The listing builds one solid part. Answer for the finished solid, in the listing's coordinates (mm). Round coordinates to 2 decimals unless told otherwise and drop trailing zeros. Order: outer loops, then holes, each group sorted by start corner. A loop starts at its lowest first (then second) coordinate and runs counter-clockwise, first axis right, second up. Notation, with made-up numbers: M 71.5,-27.75 L 80.5,-27.75 A12 ccw 80.5,-17.75 Z; hole C 21,1.5 d5. An arc over 180 degrees is marked long. Write item = value, one per line. Start each with the question number.
(1) For a pull along X with two mould halves and no side action, classify faces 1 (the face through (-1.72, 1.61, 7.76)), 2 (the face through (0, 2, -16.51)), 3 (the face through (-19.85, 1.565, -15.746)) as released by +X, released by -X, zero draft, split by the parting line, or undercut.
(2) A cutting plane is placed at A-A, the plane y = 1.8. Determine the outline of the cut face in (x, z).
(3) Straight lines are drawn through the part: probe 1 along Z at (x, y) = (0, 1.6); probe 2 along X at (y, z) = (0.7, 0); probe 3 along X at (y, z) = (1.1, -4). For each, find the intervals that lie inside material, in ascending order. Write a range as from..to.
(4) This flat-tipped pin is pushed along its axis until it touches: pin 1 (9.5 mm diameter, centred on x = 0, z = 0, fed in from -Y). Where does it stop, or does it pass through?
(5) A cutting plane is placed at B-B, the plane z = 0. Determine the outline of the cut face in (x, y) (3 decimals), and give its area (3 significant figures).
(6) A cutting plane is placed at C-C, the plane x = 0. Determine the outline of the cut face in (y, z) (3 decimals), and give its area (3 significant figures).
from build123d import *

# Parameters (mm, degrees)
BOSS_EXTRUDE1_DEPTH = 3.175
SKETCH2_R           = 7.9502
CUT_EXTRUDE1_DEPTH  = 4.175


with BuildPart() as part:
    # Sketch1 → Boss-Extrude1 (new body)
    with BuildSketch(Plane(origin=(0, 0, 0), x_dir=(1, 0, 0), z_dir=(0, 1, 0))):
        with BuildLine():
            Line((18.034, -16.51), (-18.034, -16.51))
            ThreePointArc((-18.034, -16.51), (-19.830051224, -15.766051224), (-20.574, -13.97))
            Line((-20.574, -13.97), (-20.574, 13.97))
            ThreePointArc((-20.574, 13.97), (-19.830051224, 15.766051224), (-18.034, 16.51))
            Line((-18.034, 16.51), (18.034, 16.51))
            ThreePointArc((18.034, 16.51), (19.830051224, 15.766051224), (20.574, 13.97))
            Line((20.574, 13.97), (20.574, -13.97))
            ThreePointArc((20.574, -13.97), (19.830051224, -15.766051224), (18.034, -16.51))
        make_face()
    extrude(amount=BOSS_EXTRUDE1_DEPTH)

    # Sketch2 → Cut-Extrude1 (cut, through all)
    with BuildSketch(Plane(origin=(0, 3.175, 0), x_dir=(1, 0, 0), z_dir=(0, 1, 0))):
        Circle(SKETCH2_R)
    extrude(amount=-CUT_EXTRUDE1_DEPTH, mode=Mode.SUBTRACT)


solid = part.part
Reported:
q1.face_1 = undercut
q1.face_2 = zero draft
q1.face_3 = released by -X
q2.outline = M -20.57,-13.97 A2.54 ccw -18.03,-16.51 L 18.03,-16.51 A2.54 ccw 20.57,-13.97 L 20.57,13.97 A2.54 ccw 18.03,16.51 L -18.03,16.51 A2.54 ccw -20.57,13.97 Z; hole C 0,0 d15.9
q3.probe_1 = -16.51..-7.95, 7.95..16.51
q3.probe_2 = -20.57..-7.95, 7.95..20.57
q3.probe_3 = -20.57..-6.87, 6.87..20.57
q4.pin_1 = through
q5.outline = M -20.574,0 L -7.95,0 L -7.95,3.175 L -20.574,3.175 Z; M 7.95,0 L 20.574,0 L 20.574,3.175 L 7.95,3.175 Z
q5.area = 80.2 mm²
q6.outline = M 0,-16.51 L 3.175,-16.51 L 3.175,-7.95 L 0,-7.95 Z; M 0,7.95 L 3.175,7.95 L 3.175,16.51 L 0,16.51 Z
q6.area = 54.4 mm²
